Input: part model. Units: mm. Frame: model coordinates. Face numbers are marked on the shaded views. A direction names the side the tool comes from. Coordinates: 2 decimals unless noted, no trailing zeros. Loops run counter-clockwise (first coordinate to the right, second up) from the corner with the lowest first, then second, coordinate; pieces in that order, holes last.
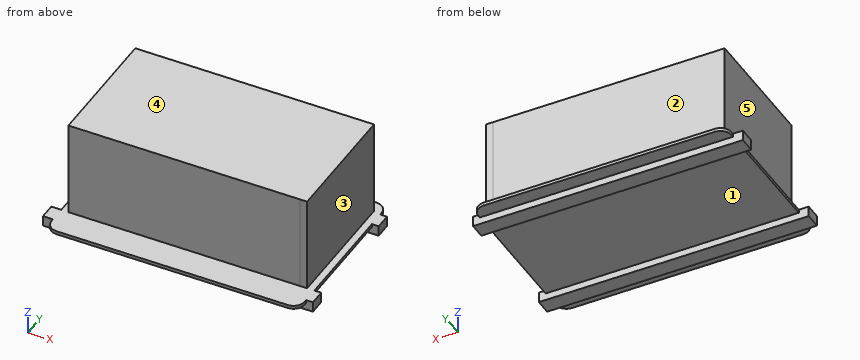
```python
from build123d import *

# Parameters (mm, degrees)
F0_W     = 123.629912734
F0_H     = 7.2298198938
F1_DEPTH = 4.826
F2_W     = 115.9501895308
F2_H     = 7.2298198938
F2_H_2   = 6.35
F2_H_3   = 63.7065680534
F3_DEPTH = 1.524
F5_R     = 5.08
F6_W     = 102.7462986398
F6_H     = 3.4007430077
F6_H_2   = 3.4007552
F7_DEPTH = 44.196
F8_DEPTH = 44.196


# Not quite as in the source:
# - ends of sketch curves that miss each other by under 0.0002 mm in the source are joined


with BuildPart() as f1:
    # F0 (on Top) → F1 (new body)
    with BuildSketch(Plane.XY):
        with Locations((-2.2894367576, -16.3875911385)):
            Rectangle(F0_W, F0_H)
    extrude(amount=F1_DEPTH)


with BuildPart() as f1b:
    # F0 (on Top) → F1, piece 2 (new body)
    with BuildSketch(Plane.XY):
        with Locations((-2.2894367576, 40.9689769149)):
            Rectangle(F0_W, F0_H)
    extrude(amount=F1_DEPTH)


with BuildPart() as f3:
    # F2 (on face) → F3 (new body)
    with BuildSketch(Plane.XY.offset(4.826)):
        with Locations((-1.5743747354, 40.9689769149)):
            Rectangle(F2_W, F2_H)
        with Locations((-1.5743747354, 47.7588868618)):
            Rectangle(F2_W, F2_H_2)
        with Locations((-1.5743747354, 5.5007829413)):
            Rectangle(F2_W, F2_H_3)
    extrude(amount=-F3_DEPTH)


with BuildPart() as f1b_1:
    add(f1b.part)

    # F4: union F3, F1
    add(f3.part)
    add(f1.part)

    # F5
    f5_edges = [f1b_1.edges().sort_by_distance(p)[0] for p in [
        (-59.54947, -26.352501, 4.064),
        (56.40072, -26.352501, 4.064),
        (56.40072, 50.933887, 4.064),
        (-59.54947, 50.933887, 4.064),
    ]]
    fillet(f5_edges, radius=F5_R)

    # F6 (on face) → F7 (join)
    with BuildSketch(Plane.XY.offset(4.826)):
        Polygon((-52.9475212097, 45.4720444977), (-56.2473237514, 45.4720444977), (-56.2473237514, -12.8244720399), (-52.9475212097, -12.8244720399), (-52.9475212097, -9.4237168399), (-52.9475212097, 42.0713014901), align=None)
        with Locations((-1.5743718898, 43.7716729939)):
            Rectangle(F6_W, F6_H)
        Polygon((53.0985676301, 45.4720334084), (49.7987774301, 45.4720334084), (49.7987774301, 42.0713014901), (49.7987774301, -9.4237168399), (49.7987774301, -12.8244717916), (53.0985676301, -12.8244717916), align=None)
        with Locations((-1.5743718898, -11.1240944399)):
            Rectangle(F6_W, F6_H_2)
    extrude(amount=F7_DEPTH)

    # F8 (add): a face of the model
    f8_faces = [f1b_1.faces().sort_by_distance(p)[0] for p in [
        (-1.5743718898, 16.3237923251, 4.826),
    ]]
    extrude(f8_faces, amount=F8_DEPTH)


solid = f1b_1.part
```
Item 1: Section query D-D (y = -16). Output: boundary loops of the cut face in (x, z), then the cut area to 3 significant figures.
Result:
outline: (-64.1, 0) - (59.53, 0) - (59.53, 4.83) - (-64.1, 4.83) - close
area: 597 mm2
Item 2: Line query: L1, parallel to Y at x = -49.5, z = 3; L2, parallel to Y at x = 22, z = 39; L3, parallel to X at y = 39.5, z = 23. Output: solid intervals per line, ascending.
Result:
L1: y = -20 to -12.77, 37.35 to 44.58
L2: y = -12.82 to 45.47
L3: x = -56.25 to 53.1
Item 3: Section query B-B (x = 18). Output: boundary loops of the cut face in (y, z).
Result:
outline: (-26.35, 3.3) - (-20, 3.3) - (-20, 0) - (-12.77, 0) - (-12.77, 3.3) - (37.35, 3.3) - (37.35, 0) - (44.58, 0) - (44.58, 3.3) - (50.93, 3.3) - (50.93, 4.83) - (45.47, 4.83) - (45.47, 49.02) - (-12.82, 49.02) - (-12.82, 4.83) - (-26.35, 4.83) - close
Item 4: Mould query, pull axis Y, two halves, no side actions, for the marked faces 1, 2 and 3. Classes: +Y half, -Y half, draft (parallel to the pull), parting line (faces both ways), or undercut.
Result:
face 1: undercut
face 2: +Y half
face 3: draft
Item 5: Reachability of the marked faces 4 and 5 from +Z, -Z, +X, -X, +Y, -Y: full face, straight path, thin tool, end or side. Return the list, or none.
Result:
face 4: +Z, +X, -X, +Y, -Y
face 5: +Z, -X, +Y, -Y
Item 6: Section query A-A (y = -4.5). Output: boundary loops of the cut face in (x, z), then the cut area to 3 significant figures.
Result:
outline: (-59.55, 3.3) - (56.4, 3.3) - (56.4, 4.83) - (53.1, 4.83) - (53.1, 49.02) - (-56.25, 49.02) - (-56.25, 4.83) - (-59.55, 4.83) - close
area: 5,010 mm2
Item 7: Contact query for flat-ended pins moving along their axis: P1, Ø1, axis at y = 45.5, z = 4, coming from the +X side; P2, Ø6, axis at y = -11, z = 42.5, coming from the +X side; P3, Ø8, axis at x = 34.5, z = 36, coming from the -Y side. Output: stop coordinate, or through.
Result:
P1: stops at x = 56.4
P2: stops at x = 53.1
P3: stops at y = -12.82
